The listing builds one solid part. Answer for the finished solid, in the listing's coordinates (mm). A direction names the side the tool comes from. Coordinates: 2 decimals unless noted, no trailing zeros. Order: outer loops, then holes, each group sorted by start corner. A loop starts at its lowest first (then second) coordinate and runs counter-clockwise, first axis right, second up. Notation, with made-up numbers: (48.5, 1.25) -> (85.5, 1.25) arc R8 cw to (85.5, 16.25) -> close; hole circle Ø8 at (71.25, 25.5). An arc over 180 degrees is marked (long way). Write item = value, one per line.
from build123d import *

# Parameters (mm, degrees)
BOSS_EXTRU_1_DEPTH                        = 12
ENL_V_MAT_EXTRU_1_DEPTH                   = 119.989845505
ENL_V_MAT_EXTRU_2_DEPTH                   = 11
ESQUISSE4_W                               = 5.5
ESQUISSE4_H                               = 3.5
ENL_V_MAT_EXTRU_3_DEPTH                   = 9.5
BOSS_EXTRU_2_DEPTH                        = 1.4
ESQUISSE13_R                              = 0.7
BOSS_EXTRU_3_DEPTH                        = 1.4
BOSS_EXTRU_6_DEPTH                        = 2.2
BOSS_EXTRU_7_DEPTH                        = 2
CHANFREIN3_SIZE                           = 2.2
CHANFREIN4_SIZE                           = 1.4
R_P_TITION_CIRCULAIRE2_COUNT              = 2
R_P_TITION_CIRCULAIRE2_ANGLE              = 120
CHANFREIN3_OF_R_P_TITION_CIRCULAIRE2_SIZE = 2.2
CHANFREIN4_OF_R_P_TITION_CIRCULAIRE2_SIZE = 1.4
ENL_V_DE_MAT_EXTRU_MINCE1_DEPTH           = 1.6
ENL_V_DE_MAT_EXTRU_MINCE1_DRAFT           = 10
ENL_V_DE_MAT_EXTRU_MINCE1_PROFILE_2_DEPTH = 1.6
ENL_V_DE_MAT_EXTRU_MINCE1_PROFILE_2_DRAFT = 10
ENL_V_DE_MAT_EXTRU_MINCE1_PROFILE_3_DEPTH = 1.6
ENL_V_DE_MAT_EXTRU_MINCE1_PROFILE_3_DRAFT = 10
ESQUISSE18_W                              = 10.5
ESQUISSE18_H                              = 2.2
ENL_V_MAT_EXTRU_10_DEPTH                  = 11


with BuildPart() as part:
    # Esquisse1 → Boss.-Extru.1 (new body)
    with BuildSketch(Plane(origin=(0, 0, 0), x_dir=(1, 0, 0), z_dir=(0, 1, 0))):
        Polygon((-77.5, -44.744645862), (77.5, -44.744645862), (0, 89.489291724), align=None)
    extrude(amount=BOSS_EXTRU_1_DEPTH)

    # Esquisse2 → Enlèv. mat.-Extru.1 (cut, through all)
    with BuildSketch(Plane(origin=(0, 12, 0), x_dir=(1, 0, 0), z_dir=(0, 1, 0))):
        Polygon((-9.237604307, 73.489291724), (9.237604307, 73.489291724), (0, 89.489291724), align=None)
        Polygon((77.5, -44.744645862), (68.262395693, -28.744645862), (59.024791386, -44.744645862), align=None)
        Polygon((-77.5, -44.744645862), (-59.024791386, -44.744645862), (-68.262395693, -28.744645862), align=None)
    extrude(amount=-ENL_V_MAT_EXTRU_1_DEPTH, mode=Mode.SUBTRACT)

    # Esquisse3 → Enlèv. mat.-Extru.2 (cut)
    with BuildSketch(Plane(origin=(0, 12, 0), x_dir=(1, 0, 0), z_dir=(0, 1, 0))):
        with BuildLine():
            Line((59.313466521, -20.244645862), (12.124355653, 61.489291724))
            ThreePointArc((12.124355653, 61.489291724), (0, 68.489291724), (-12.124355653, 61.489291724))
            Line((-12.124355653, 61.489291724), (-59.313466521, -20.244645862))
            ThreePointArc((-59.313466521, -20.244645862), (-59.313466521, -34.244645862), (-47.189110868, -41.244645862))
            Line((-47.189110868, -41.244645862), (47.189110868, -41.244645862))
            ThreePointArc((47.189110868, -41.244645862), (59.313466521, -34.244645862), (59.313466521, -20.244645862))
        make_face()
    extrude(amount=-ENL_V_MAT_EXTRU_2_DEPTH, mode=Mode.SUBTRACT)

    # Esquisse4 → Enlèv. mat.-Extru.3 (cut)
    with BuildSketch(Plane(origin=(0, 12, 0), x_dir=(1, 0, 0), z_dir=(0, 1, 0))):
        Polygon((37.093911087, 18.240753071), (34.343911087, 23.003892792), (37.375, 24.753892792), (40.125, 19.990753071), align=None)
        with Locations((0, -42.994645862)):
            Rectangle(ESQUISSE4_W, ESQUISSE4_H)
        Polygon((-37.375, 24.753892792), (-34.343911087, 23.003892792), (-37.093911087, 18.240753071), (-40.125, 19.990753071), align=None)
    extrude(amount=-ENL_V_MAT_EXTRU_3_DEPTH, mode=Mode.SUBTRACT)

    # Esquisse12 → Boss.-Extru.2 (add)
    with BuildSketch(Plane(origin=(0, 1, 0), x_dir=(1, 0, 0), z_dir=(0, 1, 0))):
        Polygon((23.928401161, 16.64408517), (28.028401161, 9.542676859), (33.397758664, 12.642676859), (29.297758664, 19.74408517), align=None)
    boss_extru_2 = extrude(amount=BOSS_EXTRU_2_DEPTH)

    # Esquisse13 → Boss.-Extru.3 (add)
    with BuildSketch(Plane(origin=(0, 2.4, 0), x_dir=(1, 0, 0), z_dir=(0, 1, 0))):
        with Locations(Location((26.364041807, 15.625431822, 0), (0, 0, 90))):
            Circle(ESQUISSE13_R)
        with Locations(Location((28.364041807, 12.161330207, 0), (0, 0, 90))):
            Circle(ESQUISSE13_R)
    boss_extru_3 = extrude(amount=BOSS_EXTRU_3_DEPTH)

    # Esquisse14 → Boss.-Extru.6 (add)
    with BuildSketch(Plane(origin=(0, 1, 0), x_dir=(1, 0, 0), z_dir=(0, 1, 0))):
        Polygon((32.699295844, 24.65244995), (37.699295844, 15.992195912), (35.967245037, 14.992195912), (30.967245037, 23.65244995), align=None)
    boss_extru_6 = extrude(amount=BOSS_EXTRU_6_DEPTH)

    # Esquisse15 → Boss.-Extru.7 (add)
    with BuildSketch(Plane(origin=(0, 3.2, 0), x_dir=(1, 0, 0), z_dir=(0, 1, 0))):
        Polygon((34.899295844, 20.841938173), (35.499295844, 19.802707689), (33.767245037, 18.802707689), (33.167245037, 19.841938173), align=None)
    boss_extru_7 = extrude(amount=BOSS_EXTRU_7_DEPTH)

    # Chanfrein3
    chanfrein3_edges = [part.edges().sort_by_distance(p)[0] for p in [
        (33.467245037, 1, -19.322322931),
        (36.833270441, 1, -15.492195912),
        (31.833270441, 1, -24.15244995),
    ]]
    chamfer(chanfrein3_edges, length=CHANFREIN3_SIZE - 0.0001)  # a hair under: the kernel refuses the full size

    # Chanfrein4
    chanfrein4_edges = [part.edges().sort_by_distance(p)[0] for p in [
        (26.613079912, 1, -18.19408517),
        (25.978401161, 1, -13.093381015),
        (30.713079912, 1, -11.092676859),
    ]]
    chamfer(chanfrein4_edges, length=CHANFREIN4_SIZE - 0.0001)  # a hair under: the kernel refuses the full size

    # Répétition circulaire2: Boss.-Extru.2, Boss.-Extru.3, Boss.-Extru.6, Boss.-Extru.7 ×2 about axis
    r_p_tition_circulaire2_axis = Axis((0, 0, 0), (0, 1, 0))
    add([boss_extru_2.rotate(r_p_tition_circulaire2_axis, i * R_P_TITION_CIRCULAIRE2_ANGLE / (R_P_TITION_CIRCULAIRE2_COUNT - 1)) for i in range(1, R_P_TITION_CIRCULAIRE2_COUNT)])
    add([boss_extru_3.rotate(r_p_tition_circulaire2_axis, i * R_P_TITION_CIRCULAIRE2_ANGLE / (R_P_TITION_CIRCULAIRE2_COUNT - 1)) for i in range(1, R_P_TITION_CIRCULAIRE2_COUNT)])
    add([boss_extru_6.rotate(r_p_tition_circulaire2_axis, i * R_P_TITION_CIRCULAIRE2_ANGLE / (R_P_TITION_CIRCULAIRE2_COUNT - 1)) for i in range(1, R_P_TITION_CIRCULAIRE2_COUNT)])
    add([boss_extru_7.rotate(r_p_tition_circulaire2_axis, i * R_P_TITION_CIRCULAIRE2_ANGLE / (R_P_TITION_CIRCULAIRE2_COUNT - 1)) for i in range(1, R_P_TITION_CIRCULAIRE2_COUNT)])

    # Chanfrein3 of Répétition circulaire2
    chanfrein3_of_r_p_tition_circulaire2_edges = [part.edges().sort_by_distance(p)[0] for p in [
        (-33.467245037, 1, -19.322322931),
        (-31.833270441, 1, -24.15244995),
        (-36.833270441, 1, -15.492195912),
    ]]
    chamfer(chanfrein3_of_r_p_tition_circulaire2_edges, length=CHANFREIN3_OF_R_P_TITION_CIRCULAIRE2_SIZE - 0.0001)  # a hair under: the kernel refuses the full size

    # Chanfrein4 of Répétition circulaire2
    chanfrein4_of_r_p_tition_circulaire2_edges = [part.edges().sort_by_distance(p)[0] for p in [
        (-29.063079912, 1, -13.950560692),
        (-24.328401161, 1, -15.951264847),
        (-24.963079912, 1, -21.051969003),
    ]]
    chamfer(chanfrein4_of_r_p_tition_circulaire2_edges, length=CHANFREIN4_OF_R_P_TITION_CIRCULAIRE2_SIZE - 0.0001)  # a hair under: the kernel refuses the full size


with BuildPart() as enl_v_de_mat_extru_mince1_tool:
    # Esquisse17 → Enlèv. de mat.-Extru.-Mince1 (with draft: the straight prism first)
    with BuildSketch(Plane(origin=(0, 12, 0), x_dir=(1, 0, 0), z_dir=(0, 1, 0))):
        Polygon((37.375, 24.753892792), (9.237604307, 73.489291724), (-9.237604307, 73.489291724), (-37.375, 24.753892792), (-35.729551733, 23.803892792), (-8.140638796, 71.589291724), (8.140638796, 71.589291724), (35.729551733, 23.803892792), align=None)
    extrude(amount=-ENL_V_DE_MAT_EXTRU_MINCE1_DEPTH)
    # Enlèv. de mat.-Extru.-Mince1: the draft: its side faces are tilted about the plane it starts from
    enl_v_de_mat_extru_mince1_sides = [enl_v_de_mat_extru_mince1_tool.faces().sort_by_distance(p)[0] for p in [
        (23.306302154, 11.2, -49.121592258),
        (0, 11.2, -73.489291724),
        (-23.306302154, 11.2, -49.121592258),
        (-36.552275866, 11.2, -24.278892792),
        (-21.935095264, 11.2, -47.696592258),
        (0, 11.2, -71.589291724),
        (21.935095264, 11.2, -47.696592258),
        (36.552275866, 11.2, -24.278892792),
    ]]
    draft(enl_v_de_mat_extru_mince1_sides, Plane(origin=(0, 12, 0), x_dir=(1, 0, 0), z_dir=(0, 1, 0)), ENL_V_DE_MAT_EXTRU_MINCE1_DRAFT)


with BuildPart() as part_1:
    add(part.part)

    # Enlèv. de mat.-Extru.-Mince1: cut by enl_v_de_mat_extru_mince1_tool
    add(enl_v_de_mat_extru_mince1_tool.part, mode=Mode.SUBTRACT)


with BuildPart() as enl_v_de_mat_extru_mince1_profile_2_tool:
    # Esquisse17 → Enlèv. de mat.-Extru.-Mince1 profile 2 (with draft: the straight prism first)
    with BuildSketch(Plane(origin=(0, 12, 0), x_dir=(1, 0, 0), z_dir=(0, 1, 0))):
        Polygon((-40.125, 19.990753071), (-68.262395693, -28.744645862), (-59.024791386, -44.744645862), (-2.75, -44.744645862), (-2.75, -42.844645862), (-57.927825874, -42.844645862), (-66.06846467, -28.744645862), (-38.479551733, 19.040753071), align=None)
    extrude(amount=-ENL_V_DE_MAT_EXTRU_MINCE1_PROFILE_2_DEPTH)
    # Enlèv. de mat.-Extru.-Mince1 profile 2: the draft: its side faces are tilted about the plane it starts from
    enl_v_de_mat_extru_mince1_profile_2_sides = [enl_v_de_mat_extru_mince1_profile_2_tool.faces().sort_by_distance(p)[0] for p in [
        (-54.193697846, 11.2, 4.376946396),
        (-63.643593539, 11.2, 36.744645862),
        (-30.887395693, 11.2, 44.744645862),
        (-2.75, 11.2, 43.794645862),
        (-30.338912937, 11.2, 42.844645862),
        (-61.998145272, 11.2, 35.794645862),
        (-52.274008201, 11.2, 4.851946396),
        (-39.302275866, 11.2, -19.515753071),
    ]]
    draft(enl_v_de_mat_extru_mince1_profile_2_sides, Plane(origin=(0, 12, 0), x_dir=(1, 0, 0), z_dir=(0, 1, 0)), ENL_V_DE_MAT_EXTRU_MINCE1_PROFILE_2_DRAFT)


with BuildPart() as part_2:
    add(part_1.part)

    # Enlèv. de mat.-Extru.-Mince1 profile 2: cut by enl_v_de_mat_extru_mince1_profile_2_tool
    add(enl_v_de_mat_extru_mince1_profile_2_tool.part, mode=Mode.SUBTRACT)


with BuildPart() as enl_v_de_mat_extru_mince1_profile_3_tool:
    # Esquisse17 → Enlèv. de mat.-Extru.-Mince1 profile 3 (with draft: the straight prism first)
    with BuildSketch(Plane(origin=(0, 12, 0), x_dir=(1, 0, 0), z_dir=(0, 1, 0))):
        Polygon((2.75, -44.744645862), (59.024791386, -44.744645862), (68.262395693, -28.744645862), (40.125, 19.990753071), (38.479551733, 19.040753071), (66.06846467, -28.744645862), (57.927825874, -42.844645862), (2.75, -42.844645862), align=None)
    extrude(amount=-ENL_V_DE_MAT_EXTRU_MINCE1_PROFILE_3_DEPTH)
    # Enlèv. de mat.-Extru.-Mince1 profile 3: the draft: its side faces are tilted about the plane it starts from
    enl_v_de_mat_extru_mince1_profile_3_sides = [enl_v_de_mat_extru_mince1_profile_3_tool.faces().sort_by_distance(p)[0] for p in [
        (30.887395693, 11.2, 44.744645862),
        (63.643593539, 11.2, 36.744645862),
        (54.193697846, 11.2, 4.376946396),
        (39.302275866, 11.2, -19.515753071),
        (52.274008201, 11.2, 4.851946396),
        (61.998145272, 11.2, 35.794645862),
        (30.338912937, 11.2, 42.844645862),
        (2.75, 11.2, 43.794645862),
    ]]
    draft(enl_v_de_mat_extru_mince1_profile_3_sides, Plane(origin=(0, 12, 0), x_dir=(1, 0, 0), z_dir=(0, 1, 0)), ENL_V_DE_MAT_EXTRU_MINCE1_PROFILE_3_DRAFT)


with BuildPart() as part_3:
    add(part_2.part)

    # Enlèv. de mat.-Extru.-Mince1 profile 3: cut by enl_v_de_mat_extru_mince1_profile_3_tool
    add(enl_v_de_mat_extru_mince1_profile_3_tool.part, mode=Mode.SUBTRACT)

    # Esquisse18 → Enlèv. mat.-Extru.10 (cut)
    with BuildSketch(Plane(origin=(0, 12, 0), x_dir=(1, 0, 0), z_dir=(0, 1, 0))):
        with Locations((37.5, -42.944645862)):
            Rectangle(ESQUISSE18_W, ESQUISSE18_H)
        with Locations((-37.5, -42.944645862)):
            Rectangle(ESQUISSE18_W, ESQUISSE18_H)
        Polygon((-52.363526329, -7.006996341), (-57.613526329, -16.100263081), (-59.518782217, -15.000263081), (-54.268782217, -5.906996341), align=None)
        Polygon((-20.113526329, 48.851642203), (-22.018782217, 49.951642203), (-16.768782217, 59.044908943), (-14.863526329, 57.944908943), align=None)
        Polygon((20.113526329, 48.851642203), (14.863526329, 57.944908943), (16.768782217, 59.044908943), (22.018782217, 49.951642203), align=None)
        Polygon((52.363526329, -7.006996341), (54.268782217, -5.906996341), (59.518782217, -15.000263081), (57.613526329, -16.100263081), align=None)
    extrude(amount=-ENL_V_MAT_EXTRU_10_DEPTH, mode=Mode.SUBTRACT)


solid = part_3.part
Q1. Section A-A, the plane y = 8.75 is taken. Give the number of separate pieces and of enclosed holes in the cut face, plus the area to 3 significant figures.
The answers:
separate_pieces = 3
enclosed_holes = 6
area = 1,330 mm2
Q2. Each of these flat-tipped pins is pushed along its axis until it touches: pin 1 Ø1.8 at (x, z) = (-40, 43.5) entering from +Y; pin 2 Ø2 at (x, y) = (24, 3.5) entering from -Z; pin 3 Ø1 at (y, z) = (6, 2) entering from +X. Where does it stop, or does it pass through?
The answers:
pin_1 = 10.4
pin_2 = -49.65
pin_3 = 53.11
Q3. The mould has two halves that part along Y. Classify faces 1 (the face through (61.935, 11.211, 35.626)), 2 (the face through (19.36, 5.77, -54.56)), 3 (the face through (-45.837, 11.211, -6.019)), 4 (the face through (-1, 1, -2)): released by +Y, released by -Y, zero draft, split by the parting line, or undercut.
The answers:
face_1 = undercut
face_2 = zero draft
face_3 = undercut
face_4 = released by +Y
Q4. Section B-B, the plane z = -29.5 is taken. Give the vertices of the cut face in (x, y).
The answers:
outline = (-34.63, 0) -> (34.63, 0) -> (34.63, 10.4) -> (32.12, 10.4) -> (32.44, 12) -> (30.59, 12) -> (30.59, 1) -> (-30.59, 1) -> (-30.59, 12) -> (-32.44, 12) -> (-32.12, 10.4) -> (-34.63, 10.4) -> close
Q5. Section D-D, the plane z = 13 is taken. Give the vertices of the cut face in (x, y).
The answers:
outline = (-59.17, 0) -> (59.17, 0) -> (59.17, 10.4) -> (58.36, 10.4) -> (58.36, 1) -> (55.82, 1) -> (55.82, 12) -> (55.13, 12) -> (55.13, 1) -> (-55.13, 1) -> (-55.13, 12) -> (-55.82, 12) -> (-55.82, 1) -> (-58.36, 1) -> (-58.36, 10.4) -> (-59.17, 10.4) -> close
Q6. Find the intervals of material crossed by line 1 along Z through (x, y) = (-16, 9.25); line 2 along Z through (x, y) = (53, 5.25); line 3 along X through (y, z) = (1.25, -17.5), in increasing order.
The answers:
line_1 = -61.78 to -58.6, -55.98 to -54.78, 41.24 to 44.74
line_2 = 2.31 to 6.64, 8.11 to 9.31, 39.98 to 44.74
line_3 = -41.56 to -37.52, -36.83 to -32.27, -30.59 to -22.11, 23.11 to 30.59, 32.27 to 36.83, 37.52 to 41.56
Q7. A tool of negligible diameter and unlimited length cuts with its end or side. For faces 5 (the face through (-35.9, 6.3, -23.9)), 6 (the face through (44, 12, 42)), 7 (the face through (29, 2.4, -15)), 8 (the face through (35.838, 6.261, -23.867)), 9 (the face through (2.75, 6, 43)), from which of +Z, -Z, +X, -X, +Y, -Y can it reach the whole face along a straight path? Write none if from no direction.
The answers:
face_5 = -X, +Y
face_6 = +Z, -Z, +X, -X, +Y
face_7 = +Y
face_8 = +X, +Y
face_9 = +Z, +Y
Q8. Section C-C, the plane z = -56 is taken. Give the vertices of the cut face in (x, y), plus the area to 3 significant figures.
The answers:
outline = (-19.34, 0) -> (19.34, 0) -> (19.34, 10.4) -> (18.53, 10.4) -> (18.53, 1) -> (15.99, 1) -> (15.99, 12) -> (15.29, 12) -> (15.29, 1) -> (-15.29, 1) -> (-15.29, 12) -> (-15.99, 12) -> (-15.99, 1) -> (-18.53, 1) -> (-18.53, 10.4) -> (-19.34, 10.4) -> close
area = 69.1 mm2
